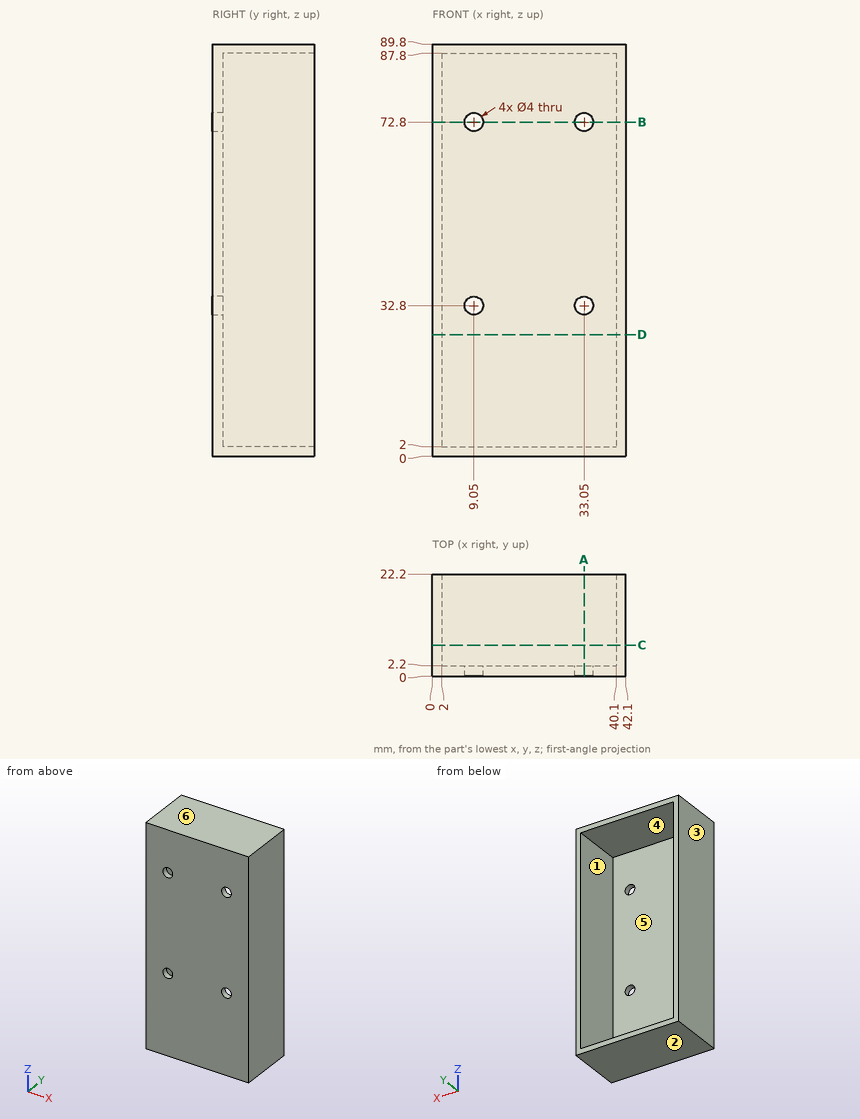
Job drawing, mm, ordinate dimensions from the low corner. One solid piece. A direction names the side the tool comes from. Coordinates: 2 decimals unless noted, no trailing zeros. Write each loop counter-clockwise with the first axis right and the second up, starting at its lowest first coordinate (ties: lowest second). Pieces come first, ordered by that corner, then holes. Notation, with made-up numbers: (9.5, 36.25) - (59.5, 36.25) arc R16 ccw to (59.5, 53.25) - close; hole circle Ø9 at (29.25, 71). An arc over 180 degrees is marked (long way). Use a Markdown table: item, result. Add a question column.
Item 1: Mould opens along X. For the marked faces 1, 2, 3 and 4 say: pulls with the +X half, pulls with the -X half, needs draft (parallel to the pull), parting line crosses it, or undercut.
Item 2: Band-saw the part on B-B, the plane z = 72.8. Give the cut face in (x, y).
Item 3: 3-axis set-ups, long thin cutter, end or side, ignore diameter. For the marked faces 5 and 6: which of +Z, -Z, +X, -X, +Y, -Y reach the whole face in a straight line?
Item 4: Flat gauge pin, fed straight in: pin 1 (6.5 mm diameter, centred on x = 9.05, z = 72.8, fed in from +Y). Where does the tip first touch, or does it go through?
Item 5: Band-saw the part on A-A, the plane x = 33.05. Give the cut face in (y, z), and give its area (3 significant figures).
Item 6: Band-saw the part on D-D, the plane z = 26.5. Give the cut face in (x, y).
Item 7: Drill centre lines: L1, parallel to X at y = 1.6, z = 32.8; L2, parallel to Z at x = 19, y = 10.5; L3, parallel to X at y = 7.25, z = 28.5. Where is each one in solid material? Low to high. Write a range as from..to.
Item 8: Band-saw the part on C-C, the plane y = 6.75. Give the cut face in (x, z).
Numbers:
| question | item | result |
|---|---|---|
| 1 | face 1 | undercut |
| 1 | face 2 | needs draft |
| 1 | face 3 | pulls with the -X half |
| 1 | face 4 | undercut |
| 2 | outline | (0, 0) - (7.05, 0) - (7.05, 2.2) - (2, 2.2) - (2, 22.2) - (0, 22.2) - close; (11.05, 0) - (31.05, 0) - (31.05, 2.2) - (11.05, 2.2) - close; (35.05, 0) - (42.1, 0) - (42.1, 22.2) - (40.1, 22.2) - (40.1, 2.2) - (35.05, 2.2) - close |
| 3 | face 5 | +Y |
| 3 | face 6 | +Z, +X, -X, +Y, -Y |
| 4 | pin 1 | y = 2.2 |
| 5 | outline | (0, 0) - (22.2, 0) - (22.2, 2) - (2.2, 2) - (2.2, 30.8) - (0, 30.8) - close; (0, 34.8) - (2.2, 34.8) - (2.2, 70.8) - (0, 70.8) - close; (0, 74.8) - (2.2, 74.8) - (2.2, 87.8) - (22.2, 87.8) - (22.2, 89.8) - (0, 89.8) - close |
| 5 | area | 260 mm2 |
| 6 | outline | (0, 0) - (42.1, 0) - (42.1, 22.2) - (40.1, 22.2) - (40.1, 2.2) - (2, 2.2) - (2, 22.2) - (0, 22.2) - close |
| 7 | L1 | 0..7.05, 11.05..31.05, 35.05..42.1 |
| 7 | L2 | 0..2, 87.8..89.8 |
| 7 | L3 | 0..2, 40.1..42.1 |
| 8 | outline | (0, 0) - (42.1, 0) - (42.1, 89.8) - (0, 89.8) - close; hole (2, 2) - (40.1, 2) - (40.1, 87.8) - (2, 87.8) - close |
